Input: dimensioned drawing with shaded views. Units: mm. Origin: part minimum x, y, z. A direction names the side the tool comes from. Give positions to 0.01 mm unless a question says otherwise; leave off trailing zeros. Order: outer loops, then holes, each group sorted by start corner. A loop starts at its lowest first (then second) coordinate and runs counter-clockwise, first axis right, second up. Notation, with made-up numbers: (-5.75, 35.5) -> (15.25, 35.5) arc R27 cw to (15.25, 69.5) -> close; hole circle Ø8 at (59.25, 27). An arc over 180 degrees is marked (long way). One line per question, with ' | ' between items. Start each with the question number.
(1) Section C-C (x = 14.5). Return loops of the section in (y, z).
(2) Ray query, L1, parallel to Y at x = 33, z = 4.2; L2, parallel to X at y = 47.5, z = 2.65; L3, parallel to X at y = 31, z = 0.55. Return the intervals inside material, ascending.
(3) First-contact query: pin 1 Ø6 at (x, y) = (49.78, 19.05) entering from +Z; pin 2 Ø1.5 at (y, z) = (26, 1.5) entering from -X; pin 3 Ø1.5 at (x, z) = (7, 2.5) entering from -Y; pin 4 Ø1.5 at (x, z) = (46, 2) entering from +Y. Flat tips, straight axial feed; report the tip coordinate or a pass-through.
(4) Mould query, pull axis X, two halves, no side actions, for the marked faces 6 and 7. Classes: +X half, -X half, draft (parallel to the pull), parting line (faces both ways), or undercut.
(5) Section B-B (z = 4.3). State how many separate pieces and enclosed holes the cut face has, then the cut area to 4 significant figures.
(6) Set-up query: the marked faces 1, 2, 3, 4 and 5. Return all of +Z, -Z, +X, -X, +Y, -Y with unobstructed straight access to the full face (end or side cutting, diameter ignored); none if empty.
(7) Section A-A (y = 19.05). Return loops of the section in (x, z).
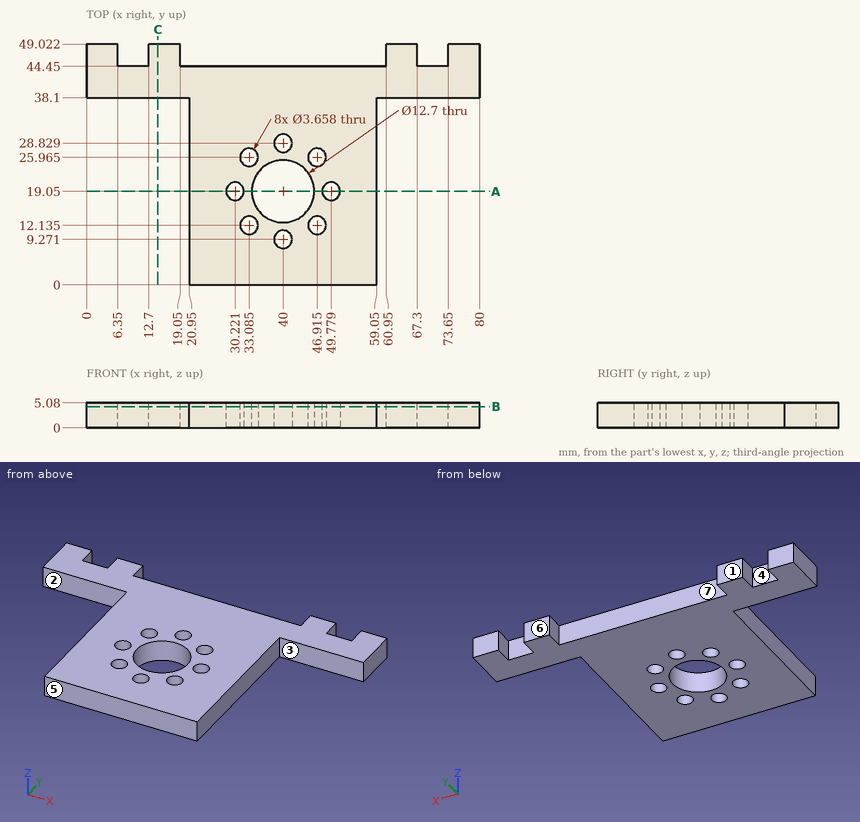
Response:
1) outline: (38.1, 0) -> (49.02, 0) -> (49.02, 5.08) -> (38.1, 5.08) -> close
2) L1: y = 0 to 10.31, 13.96 to 24.14, 27.79 to 44.45 | L2: x = 0 to 6.35, 12.7 to 19.05, 60.95 to 67.3, 73.65 to 80 | L3: x = 20.95 to 59.05
3) pin 1: stops at z = 5.08 | pin 2: stops at x = 20.95 | pin 3: stops at y = 38.1 | pin 4: stops at y = 44.45
4) face 6: draft | face 7: undercut
5) separate pieces: 1 | enclosed holes: 9 | area: 1,865 mm^2
6) face 1: +Z, -Z, +X, -X, +Y | face 2: +Z, -Z, -X, -Y | face 3: +Z, -Z, +X, -Y | face 4: +Z, -Z, +Y | face 5: +Z, -Z, +X, -X, -Y
7) outline: (20.95, 0) -> (28.39, 0) -> (28.39, 5.08) -> (20.95, 5.08) -> close; (32.05, 0) -> (33.65, 0) -> (33.65, 5.08) -> (32.05, 5.08) -> close; (46.35, 0) -> (47.95, 0) -> (47.95, 5.08) -> (46.35, 5.08) -> close; (51.61, 0) -> (59.05, 0) -> (59.05, 5.08) -> (51.61, 5.08) -> close
